```python
from build123d import *

# Parameters (mm, degrees)
SKETCH1_R           = 5
BOSS_EXTRUDE1_DEPTH = 12
SKETCH2_R           = 25
BOSS_EXTRUDE2_DEPTH = 50
SKETCH3_R           = 20
CUT_EXTRUDE1_DEPTH  = 63
FILLET1_R           = 3
CHAMFER1_SIZE       = 2


with BuildPart() as part:
    # Sketch1 → Boss-Extrude1 (new body)
    with BuildSketch(Plane(origin=(0, 0, 0), x_dir=(1, 0, 0), z_dir=(0, 1, 0))):
        with BuildLine():
            Line((-90, -50), (90, -50))
            ThreePointArc((90, -50), (97.071067812, -47.071067812), (100, -40))
            Line((100, -40), (100, 40))
            ThreePointArc((100, 40), (97.071067812, 47.071067812), (90, 50))
            Line((90, 50), (-90, 50))
            ThreePointArc((-90, 50), (-97.071067812, 47.071067812), (-100, 40))
            Line((-100, 40), (-100, -40))
            ThreePointArc((-100, -40), (-97.071067812, -47.071067812), (-90, -50))
        make_face()
        with Locations((-80, -30)):
            Circle(SKETCH1_R, mode=Mode.SUBTRACT)
        with Locations((-80, 30)):
            Circle(SKETCH1_R, mode=Mode.SUBTRACT)
        with Locations((80, 30)):
            Circle(SKETCH1_R, mode=Mode.SUBTRACT)
        with Locations((80, -30)):
            Circle(SKETCH1_R, mode=Mode.SUBTRACT)
    extrude(amount=BOSS_EXTRUDE1_DEPTH)

    # Sketch2 → Boss-Extrude2 (add)
    with BuildSketch(Plane(origin=(0, 12, 0), x_dir=(1, 0, 0), z_dir=(0, 1, 0))):
        Circle(SKETCH2_R)
    extrude(amount=BOSS_EXTRUDE2_DEPTH)

    # Sketch3 → Cut-Extrude1 (cut, through all)
    with BuildSketch(Plane(origin=(0, 62, 0), x_dir=(1, 0, 0), z_dir=(0, 1, 0))):
        Circle(SKETCH3_R)
    extrude(amount=-CUT_EXTRUDE1_DEPTH, mode=Mode.SUBTRACT)

    # Fillet1
    fillet1_edges = [part.edges().sort_by_distance(p)[0] for p in [
        (-25, 12, 0),
    ]]
    fillet(fillet1_edges, radius=FILLET1_R)

    # Chamfer1
    chamfer1_edges = [part.edges().sort_by_distance(p)[0] for p in [
        (-25, 62, 0),
    ]]
    chamfer(chamfer1_edges, length=CHAMFER1_SIZE)


solid = part.part
```
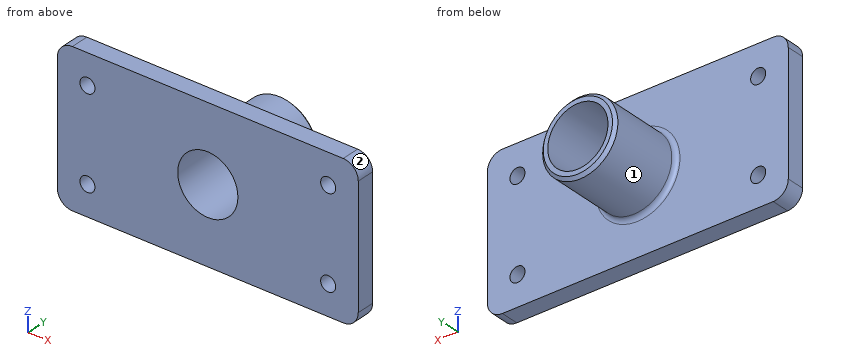
Input: part model. Units: mm. Frame: model coordinates. Face numbers are marked on the shaded views. A direction names the side the tool comes from. Give positions to 0.01 mm unless a question says otherwise; leave off trailing zeros. Loops run counter-clockwise (first coordinate to the right, second up) from the corner with the lowest first, then second, coordinate; pieces in that order, holes last. Notation, with made-up numbers: (33, -18) -> (80, -18) arc R19 cw to (80, -5) -> close; hole circle Ø6 at (21, 29). An arc over 180 degrees is marked (long way). Use a Markdown table: item, result.
Q1. Section query A-A, the plane x = 0. Return the cut outline in (y, z), plus the area to 3 significant figures.
Entries:
| item | result |
|---|---|
| outline | (0, -50) -> (12, -50) -> (12, -28) arc R3 cw to (15, -25) -> (60, -25) -> (62, -23) -> (62, -20) -> (0, -20) -> close; (0, 20) -> (62, 20) -> (62, 23) -> (60, 25) -> (15, 25) arc R3 cw to (12, 28) -> (12, 50) -> (0, 50) -> close |
| area | 1,220 mm² |
Q2. Section query D-D, the plane x = 80. Return the cut outline in (y, z), plus the area to 3 significant figures.
Entries:
| item | result |
|---|---|
| outline | (0, -50) -> (12, -50) -> (12, -35) -> (0, -35) -> close; (0, -25) -> (12, -25) -> (12, 25) -> (0, 25) -> close; (0, 35) -> (12, 35) -> (12, 50) -> (0, 50) -> close |
| area | 960 mm² |
Q3. Ray query, probe 1 along X at (y, z) = (7.75, 30); probe 2 along Z at (x, y) = (-80, 9); probe 3 along X at (y, z) = (4.5, 33). Return the intervals inside material, ascending. Write a range as from..to.
Entries:
| item | result |
|---|---|
| probe 1 | x = -100..-85, -75..75, 85..100 |
| probe 2 | z = -50..-35, -25..25, 35..50 |
| probe 3 | x = -100..-84, -76..76, 84..100 |
Q4. Section query B-B, the plane z = -30. Return the cut outline in (x, y).
Entries:
| item | result |
|---|---|
| outline | (-100, 0) -> (-85, 0) -> (-85, 12) -> (-100, 12) -> close; (-75, 0) -> (75, 0) -> (75, 12) -> (-75, 12) -> close; (85, 0) -> (100, 0) -> (100, 12) -> (85, 12) -> close |
Q5. Section query C-C, the plane z = 0. Return the cut outline in (x, y).
Entries:
| item | result |
|---|---|
| outline | (-100, 0) -> (-20, 0) -> (-20, 62) -> (-23, 62) -> (-25, 60) -> (-25, 15) arc R3 cw to (-28, 12) -> (-100, 12) -> close; (20, 0) -> (100, 0) -> (100, 12) -> (28, 12) arc R3 cw to (25, 15) -> (25, 60) -> (23, 62) -> (20, 62) -> close |
Q6. First-contact query: P1, Ø6, axis at x = 30.5, z = 0, coming from the +Y side; P2, Ø3, axis at y = 50.5, z = 20.5, coming from the -X side; P3, Ø8, axis at y = 26, z = 18, coming from the +X side. Flat tips, straight axial feed; report the tip coordinate or a pass-through.
Entries:
| item | result |
|---|---|
| P1 | stops at y = 12.04 |
| P2 | stops at x = -16.25 |
| P3 | stops at x = 20.71 |
Q7. Access query for the marked faces 1 and 2. Directions: +Z, -Z, +X, -X, +Y, -Y. A direction counts if a zero-diameter tool reaches every point of the face in a straight line with its end or side. Return the directions, or none.
Entries:
| item | result |
|---|---|
| face 1 | +Y |
| face 2 | +Z, +X, +Y, -Y |
